Check sheet for the drawn part. Datum: minimum x, y, z corner. Units: mm. A direction names the side the tool comes from. Round coordinates to 2 decimals unless told otherwise and drop trailing zeros. Write each loop counter-clockwise with the first axis right and the second up, starting at its lowest first coordinate (ties: lowest second). Pieces come first, ordered by that corner, then holes. Notation, with made-up numbers: (-28, -2.75) - (12, -2.75) arc R12 cw to (12, 17.25) - close; hole circle Ø8 at (46.25, -36). An arc over 180 degrees is marked (long way). Answer as a JSON object with one key per item and string values.
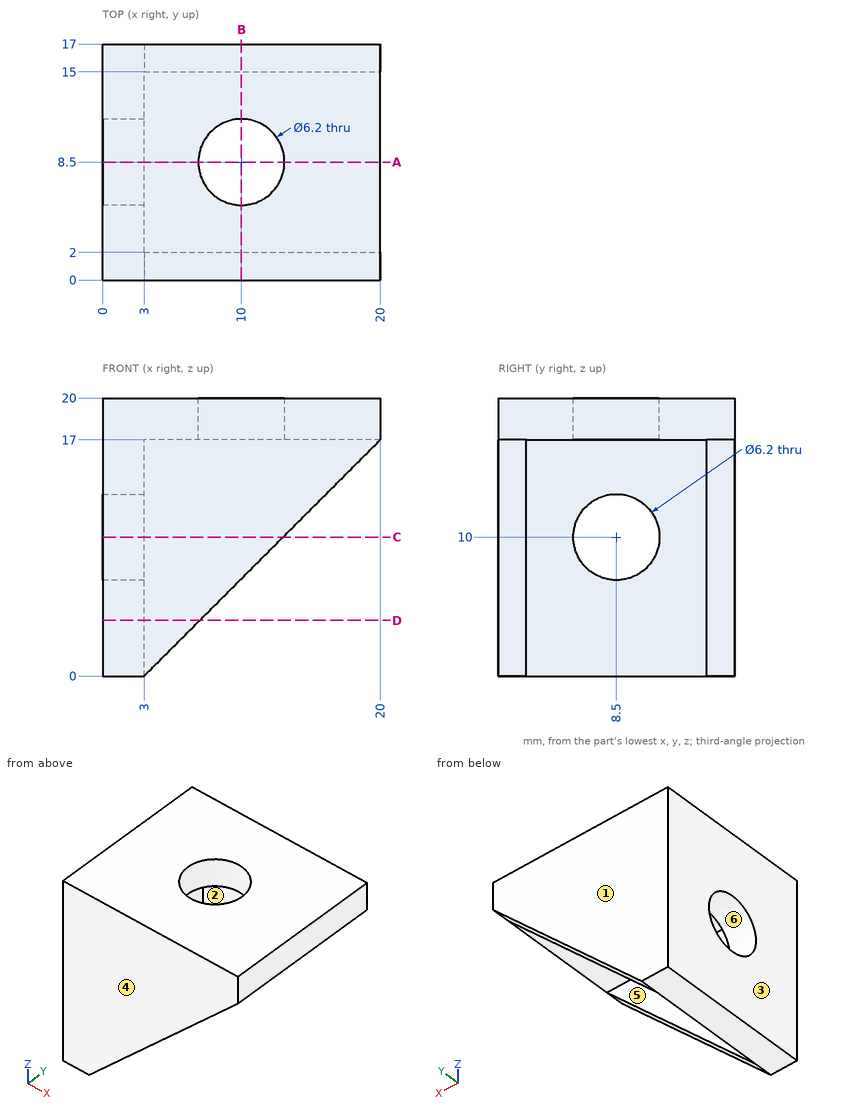
Q1. Set-up check for the marked faces 5 and 6: record each of +Z, -Z, +X, -X, +Y, -Y from which the full face is reachable in a straight line by a thin tool's end or side.
Geometry check:
{"face 5": "-Z, +X", "face 6": "+X, -X"}
Q2. Section check A-A, the plane y = 8.5. Record the cut outline in (x, z).
Geometry check:
{"outline": "(0, 0) - (3, 0) - (3, 6.9) - (0, 6.9) - close; (0, 13.1) - (3, 13.1) - (3, 17) - (6.9, 17) - (6.9, 20) - (0, 20) - close; (13.1, 17) - (20, 17) - (20, 20) - (13.1, 20) - close"}
Q3. Gauge pin test, flat end, axial feed: P1, Ø8, axis at y = 6.5, z = 4, coming from the +X side. Record the tip position at first contact, or that the pin passes through.
Geometry check:
{"P1": "stops at x = 3"}
Q4. Section check B-B, the plane x = 10. Record the cut outline in (y, z).
Geometry check:
{"outline": "(0, 7) - (2, 7) - (2, 17) - (5.4, 17) - (5.4, 20) - (0, 20) - close; (11.6, 17) - (15, 17) - (15, 7) - (17, 7) - (17, 20) - (11.6, 20) - close"}
Q5. Section check C-C, the plane z = 10. Record the cut outline in (x, y), then the cut area to 3 significant figures.
Geometry check:
{"outline": "(0, 0) - (13, 0) - (13, 2) - (3, 2) - (3, 5.4) - (0, 5.4) - close; (0, 11.6) - (3, 11.6) - (3, 15) - (13, 15) - (13, 17) - (0, 17) - close", "area": "72.4 mm2"}
Q6. Material ranges on line 1 along Y through (x, z) = (3.5, 7.75); line 2 along Y through (x, z) = (10, 17.95); line 3 along Z through (x, y) = (18.5, 9), recorded low to high. Write a range as [from, to].
Geometry check:
{"line 1": "y = [0, 2], [15, 17]", "line 2": "y = [0, 5.4], [11.6, 17]", "line 3": "z = [17, 20]"}
Q7. Release check for a two-part mould opening along Y. For the marked faces 1, 2, 3 and 4 record: released by +Y, released by -Y, zero draft, split by the parting line, or undercut.
Geometry check:
{"face 1": "released by +Y", "face 2": "undercut", "face 3": "zero draft", "face 4": "released by -Y"}
Q8. Section check D-D, the plane z = 4. Record the cut outline in (x, y).
Geometry check:
{"outline": "(0, 0) - (7, 0) - (7, 2) - (3, 2) - (3, 15) - (7, 15) - (7, 17) - (0, 17) - close"}
